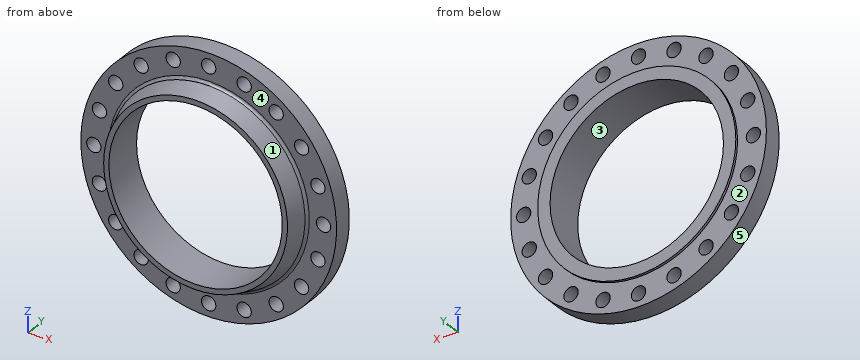
Autodesk Inventor part; units mm, degrees
ref_plane "YZ Plane" through (0, 0, 0) normal (1, 0, 0) x (0, 1, 0)
ref_plane "XZ Plane" through (0, 0, 0) normal (0, 1, 0) x (-1, 0, 0)
ref_plane "XY Plane" through (0, 0, 0) normal (0, 0, 1) x (1, 0, 0)
sketch "Sketch1" plane through (0, 0, 0) normal (0, 0, 1) x (1, 0, 0)
  line L0 (0, 94.8129) -> (0, -76.7795)
  line L1 (-200, 0) -> (-228.5, 0)
  line L2 (-228.5, 0) -> (-228.5, -6)
  line L3 (-228.5, -6) -> (-295, -6)
  line L4 (-295, -6) -> (-295, -50)
  line L5 (-295, -50) -> (-232.0453, -50)
  line L6 (-225.4045, -54.7864) -> (-212, -95)
  line L7 (-212, -95) -> (-200, -95)
  line L8 (-200, -95) -> (-200, 0)
  arc A0 (-225.4045, -54.7864) -> (-232.0453, -50) centre (-232.0453, -57) ccw
  line L9 (-228.5, -4) -> (-204, -4) construction
  line L10 (-204, 0) -> (-204, -95) construction
  point P0 (0, 0)
  point P1 (-227, -50)
  dimension "d1" = 590
  dimension "d2" = 457
  dimension "d3" = 400
  dimension "d4" = 454
  dimension "d5" = 424
  dimension "d6" = 95
  dimension "d7" = 50
  dimension "d8" = 6
  dimension "d13" = 7
  dimension "d25" = 4
  dimension "d26" = 4
revolve "Revolution1" add sketch "Sketch1" angle 360 about axis through (0, 94.8129, 0) along (0, -1, 0)
sketch "Sketch2" plane through (0, -50, 0) normal (0, -1, 0) x (1, 0, 0)
  circle A0 centre (-265, 0) radius 16.5
  point P0 (0, 0)
  dimension "d15" = 33
  dimension "d16" = 265
extrude "Extrusion1" cut sketch "Sketch2" against normal through all
pattern_circular "Circular Pattern1" count 20 over 360 about axis through (0, -28, 0) along (0, 1, 0) of "Extrusion1"
equation "\"d15\" = d_"
equation "\"d1\" = D1_"
equation "\"d2\" = D5_"
equation "\"d3\" = D"
equation "\"d5\" = D6_"
equation "\"d6\" = H_"
equation "\"d7\" = b"
equation "\"D\" = 400"
equation "\"D1_\" = 590"
equation "\"D5_\" = 457"
equation "\"D6_\" = 424"
equation "\"D7_\" = 454"
equation "\"H_\" = 95"
equation "\"b\" = 50"
equation "\"d_\" = 33"
properties part number "Flange 10-400-4,0 GOST 28759.3-90" material "Steel"
Work out the finished part from the listing and answer in its coordinate system (mm). Face numbers are marked on the shaded views. A direction names the side the tool comes from. Coordinates: 2 decimals unless noted, no trailing zeros. Write each loop counter-clockwise with the first axis right and the second up, starting at its lowest first coordinate (ties: lowest second). Pieces come first, ordered by that corner, then holes. Notation, with made-up numbers: M -11,-5 L 9,-5 A31 ccw 9,34 Z; hole C 62.5,-10 d1. An arc over 180 degrees is marked long. Write item = value, one per line.
1. The part is cut by section D-D (y = -63). Determine the outline of the cut face in (x, z).
Solution:
outline = C 0,0 d445.33; hole C 0,0 d400
2. Determine the mould class of the marked faces 3, 4 and 5 for opening direction X: released by +X, released by -X, zero draft, split by the parting line, or undercut.
Solution:
face_3 = undercut
face_4 = zero draft
face_5 = split by the parting line
3. Flat-ended cylindrical pins translate along their axes: pin 1 (2 mm diameter, centred on x = -212, y = -40, fed in from -Z) (3 decimals); pin 2 (20 mm diameter, centred on x = 81.89, z = 252.03, fed in from +Y); pin 3 (5 mm diameter, centred on x = 105, y = -46, fed in from +Z); pin 4 (4 mm diameter, centred on y = -81, z = -200.5, fed in from +X). Find the tip coordinate at first contact, or state that the pin passes through.
Solution:
pin_1 = -206.165
pin_2 = through
pin_3 = 276.62
pin_4 = 87.14
4. The part is cut by section A-A (z = 0). Determine the outline of the cut face in (x, y).
Solution:
outline = M -295,-50 L -281.5,-50 L -281.5,-6 L -295,-6 Z; M -248.5,-50 L -232.05,-50 A7 cw -225.4,-54.79 L -212,-95 L -200,-95 L -200,0 L -228.5,0 L -228.5,-6 L -248.5,-6 Z; M 200,-95 L 212,-95 L 225.4,-54.79 A7 cw 232.05,-50 L 248.5,-50 L 248.5,-6 L 228.5,-6 L 228.5,0 L 200,0 Z; M 281.5,-50 L 295,-50 L 295,-6 L 281.5,-6 Z
5. The part is cut by section B-B (x = 0). Determine the outline of the cut face in (y, z), then the cut area to 3 significant figures.
Solution:
outline = M -95,-212 L -54.79,-225.4 A7 cw -50,-232.05 L -50,-248.5 L -6,-248.5 L -6,-228.5 L 0,-228.5 L 0,-200 L -95,-200 Z; M -95,200 L 0,200 L 0,228.5 L -6,228.5 L -6,248.5 L -50,248.5 L -50,232.05 A7 cw -54.79,225.4 L -95,212 Z; M -50,-295 L -6,-295 L -6,-281.5 L -50,-281.5 Z; M -50,281.5 L -6,281.5 L -6,295 L -50,295 Z
area = 7,560 mm2
6. For the marked faces 1 and 2, determine the directions among +Z, -Z, +X, -X, +Y, -Y from which every point of the face is accessible in a straight line to the end or side of a thin tool.
Solution:
face_1 = -Y
face_2 = +Y
7. Straight lines are drawn through the part: line 1 (X direction, y = -49, z = 11); line 2 (Z direction, x = 158, y = -10.5); line 3 (X direction, y = -40, z = -265). For each, find the intervals that lie inside material, in ascending order. Write a range as from..to.
Solution:
line_1 = -294.79..-277.3, -252.7..-199.7, 199.7..252.7, 277.3..294.79
line_2 = -249.12..-230.74, -198.04..-122.62, 122.62..198.04, 230.74..249.12
line_3 = -129.61..-92.09, -71.69..-16.5, 16.5..71.69, 92.09..129.61
